The listing builds one solid part. Answer for the finished solid, in the listing's coordinates (mm). A direction names the side the tool comes from. Coordinates: 2 decimals unless noted, no trailing zeros. Loops run counter-clockwise (first coordinate to the right, second up) from the corner with the lowest first, then second, coordinate; pieces in that order, holes last. Notation, with made-up numbers: (85.5, 18) - (102.5, 18) arc R24 cw to (102.5, 48) - close; hole circle Ø7 at (-39, 19). An arc over 180 degrees is marked (long way). Write each question's results on one line, items separated by ' | '. Start each with the question number.
(1) Determine the mould class of faces 4 (the flat face through (-12.5, 3, -18)), 5 (the flat face through (0, 5, 22.5)), 6 (the flat face through (15, 1, -18)) for opening direction X: released by +X, released by -X, zero draft, split by the parting line, or undercut.
(2) Given pin 1 Ø17.5 at (x, z) = (7.5, 8.5) entering from +Y; pin 2 Ø1.6 at (x, z) = (-14.5, 18.5) entering from +Y, each flat-ended and moving along its own axis, determine where each tip first touches the part or whether it passes through.
(3) Find section A-A on x = -1. Determine the outline of the cut face in (y, z).
(4) Find section C-C on y = 4. Determine the outline of the cut face in (x, z).
(5) Find section D-D on x = -6. Determine the outline of the cut face in (y, z).
(6) Find section B-B on y = 13.25. Determine the outline of the cut face in (x, z).
(7) For faces 1 (the flat face through (-4, 7, 22)), 2 (the cylindrical face through (16.08, 3.03, -19.18)), 3 (the flat face through (0, 9, -22.5)), determine the directions among +Z, -Z, +X, -X, +Y, -Y from which every point of the face is accessible in a straight line to the end or side of a thin tool.
(8) Consider line 1 (X direction, y = 2.4, z = -18); line 2 (Z direction, x = 8, y = 3.5); line 3 (X direction, y = 5.75, z = -14.5). Determine where each line is inside the solid, lowest interval first. Write a range as from..to.
from build123d import *

# Parameters (mm, degrees)
SKETCH1_W             = 39
SKETCH1_H             = 45
BODY_DEPTH            = 18.6
SHELL1_T              = -2
SKETCH3_W             = 5
SKETCH3_H             = 5
INSERTS_SUPPORT_DEPTH = 3
SKETCH4_R             = 1.6
INSERTS_HOLES_DEPTH   = 4
USB_HOLE_REACH        = 54.452
SKETCH5_W             = 15
SKETCH5_H             = 7.5
JACK_HOLE_REACH       = 54.452
SKETCH6_R             = 4


with BuildPart() as part:
    # Sketch1 → Body (new body)
    with BuildSketch(Plane(origin=(0, 0, 0), x_dir=(1, 0, 0), z_dir=(0, 1, 0))):
        Rectangle(SKETCH1_W, SKETCH1_H)
    extrude(amount=BODY_DEPTH)

    # Shell1
    shell1_openings = [part.faces().sort_by_distance(p)[0] for p in [
        (0, 18.6, 0),
    ]]
    offset(amount=SHELL1_T, openings=shell1_openings, kind=Kind.INTERSECTION)

    # Sketch3 → Inserts_Support (add)
    with BuildSketch(Plane(origin=(0, 2, 0), x_dir=(1, 0, 0), z_dir=(0, 1, 0))):
        with Locations((-15, 18)):
            Rectangle(SKETCH3_W, SKETCH3_H)
        with Locations((15, 18)):
            Rectangle(SKETCH3_W, SKETCH3_H)
        with Locations((15, -18)):
            Rectangle(SKETCH3_W, SKETCH3_H)
        with Locations((-15, -18)):
            Rectangle(SKETCH3_W, SKETCH3_H)
    extrude(amount=INSERTS_SUPPORT_DEPTH)

    # Sketch4 → Inserts_Holes (cut)
    with BuildSketch(Plane(origin=(0, 5, 0), x_dir=(1, 0, 0), z_dir=(0, 1, 0))):
        with Locations(Location((-15, 18, 0), (0, 0, 270))):
            Circle(SKETCH4_R)
        with Locations(Location((15, 18, 0), (0, 0, 270))):
            Circle(SKETCH4_R)
        with Locations(Location((15, -18, 0), (0, 0, 270))):
            Circle(SKETCH4_R)
        with Locations(Location((-15, -18, 0), (0, 0, 270))):
            Circle(SKETCH4_R)
    extrude(amount=-INSERTS_HOLES_DEPTH, mode=Mode.SUBTRACT)

    # Sketch5 → USB_Hole (cut, up to next)
    with BuildSketch(Plane.XY.offset(22.5), mode=Mode.PRIVATE) as usb_hole_sk1:
        with Locations((-3.5, 10.75)):
            Rectangle(SKETCH5_W, SKETCH5_H)
    usb_hole_tool1 = extrude(usb_hole_sk1.sketch, amount=-USB_HOLE_REACH, mode=Mode.PRIVATE) & part.part
    add(usb_hole_tool1.solids().sort_by_distance((-3.5, 10.75, 22.5))[0], mode=Mode.SUBTRACT)

    # Sketch6 → Jack_Hole (cut, up to next)
    with BuildSketch(Plane(origin=(0, 0, -22.5), x_dir=(-1, 0, 0), z_dir=(0, 0, -1)), mode=Mode.PRIVATE) as jack_hole_sk1:
        with Locations((6, 13.25)):
            Circle(SKETCH6_R)
    jack_hole_tool1 = extrude(jack_hole_sk1.sketch, amount=-JACK_HOLE_REACH, mode=Mode.PRIVATE) & part.part
    add(jack_hole_tool1.solids().sort_by_distance((-6, 13.25, -22.5))[0], mode=Mode.SUBTRACT)


solid = part.part
Values:
1) face 4: undercut | face 5: zero draft | face 6: undercut
2) pin 1: stops at y = 5 | pin 2: stops at y = 1
3) outline: (0, -22.5) - (18.6, -22.5) - (18.6, -20.5) - (2, -20.5) - (2, 20.5) - (7, 20.5) - (7, 22.5) - (0, 22.5) - close; (14.5, 20.5) - (18.6, 20.5) - (18.6, 22.5) - (14.5, 22.5) - close
4) outline: (-19.5, -22.5) - (19.5, -22.5) - (19.5, 22.5) - (-19.5, 22.5) - close; hole (-17.5, -15.5) - (-12.5, -15.5) - (-12.5, -20.5) - (12.5, -20.5) - (12.5, -15.5) - (17.5, -15.5) - (17.5, 15.5) - (12.5, 15.5) - (12.5, 20.5) - (-12.5, 20.5) - (-12.5, 15.5) - (-17.5, 15.5) - close; hole circle Ø3.2 at (-15, -18); hole circle Ø3.2 at (-15, 18); hole circle Ø3.2 at (15, -18); hole circle Ø3.2 at (15, 18)
5) outline: (0, -22.5) - (9.25, -22.5) - (9.25, -20.5) - (2, -20.5) - (2, 20.5) - (7, 20.5) - (7, 22.5) - (0, 22.5) - close; (14.5, 20.5) - (18.6, 20.5) - (18.6, 22.5) - (14.5, 22.5) - close; (17.25, -22.5) - (18.6, -22.5) - (18.6, -20.5) - (17.25, -20.5) - close
6) outline: (-19.5, -22.5) - (-10, -22.5) - (-10, -20.5) - (-17.5, -20.5) - (-17.5, 20.5) - (-11, 20.5) - (-11, 22.5) - (-19.5, 22.5) - close; (-2, -22.5) - (19.5, -22.5) - (19.5, 22.5) - (4, 22.5) - (4, 20.5) - (17.5, 20.5) - (17.5, -20.5) - (-2, -20.5) - close
7) face 1: +Z | face 2: +Y | face 3: -Z, +X, -X, +Y, -Y
8) line 1: x = -19.5..-16.6, -13.4..-12.5, 12.5..13.4, 16.6..19.5 | line 2: z = -22.5..-20.5, 20.5..22.5 | line 3: x = -19.5..-17.5, 17.5..19.5
